Autodesk Inventor part; units mm, degrees
ref_plane "YZ Plane" through (0, 0, 0) normal (1, 0, 0) x (0, 1, 0)
ref_plane "XZ Plane" through (0, 0, 0) normal (0, 1, 0) x (-1, 0, 0)
ref_plane "XY Plane" through (0, 0, 0) normal (0, 0, 1) x (1, 0, 0)
sketch "Sketch1" plane through (0, 0, 0) normal (0, 1, 0) x (-1, 0, 0)
  line L0 (0, 0) -> (0, -650)
  line L1 (0, -650) -> (650, -650)
  line L2 (650, -647) -> (650, -3)
  line L3 (650, 0) -> (0, 0)
  line L4 (0, 0) -> (3, 0)
  line L5 (3, -3) -> (3, -647)
  line L6 (3, -650) -> (0, -650)
  line L7 (0, -650) -> (0, -647)
  line L8 (650, -647) -> (650, -650)
  line L9 (650, -650) -> (647, -650)
  line L10 (647, -647) -> (647, -3)
  line L11 (647, 0) -> (650, 0)
  line L12 (650, 0) -> (650, -3)
  line L13 (0, -3) -> (0, 0)
  line L14 (0, 0) -> (0, -37)
  line L15 (650, -37) -> (650, 0)
  line L16 (650, 0) -> (613, 0)
  line L17 (613, -3) -> (613, -647)
  line L18 (613, -650) -> (650, -650)
  line L19 (650, -650) -> (650, -613)
  line L20 (0, -613) -> (0, -650)
  line L21 (0, -650) -> (37, -650)
  line L22 (37, 0) -> (0, 0)
  line L23 (3, -147.3087) -> (3, -94.9828)
  line L24 (147.3087, -3) -> (94.9828, -3)
  circle A0 centre (16.1109, -108.0348) radius 3
  line L25 (0, -650) -> (3, -650)
  line L26 (0, -647) -> (0, -650)
  line L27 (0, -650) -> (0, -613)
  line L28 (37, -650) -> (0, -650)
  line L29 (3, -502.6913) -> (3, -555.0172)
  line L30 (147.3087, -647) -> (94.9828, -647)
  circle A1 centre (16.1109, -541.9652) radius 3
  line L31 (37, -650) -> (37, -37)
  line L32 (37, -3) -> (37, 0)
  line L33 (650, -3) -> (34.9546, -3)
  line L34 (34.9546, -647) -> (650, -647)
  line L35 (37, -37) -> (0, 0)
  line L36 (37, -613) -> (0, -650)
  line L37 (0, -650) -> (3, -647)
  line L38 (3, -647) -> (3, -3)
  line L39 (3, -3) -> (0, 0)
  line L40 (3, -325) -> (3, -458)
  line L41 (3, -458) -> (20, -458)
  line L42 (3, -325) -> (3, -192)
  line L43 (3, -192) -> (20, -192)
  circle A2 centre (20, -192) radius 3
  circle A3 centre (20, -458) radius 3
  line L44 (647, -3) -> (630, -3)
  line L45 (630, -3) -> (630, -20)
  line L46 (647, -647) -> (630, -647)
  line L47 (630, -647) -> (630, -630)
  circle A4 centre (630, -630) radius 3
  circle A5 centre (630, -20) radius 3
  point P0 (37, -647)
  dimension "d0" = 650
  dimension "d1" = 650
  dimension "d2" = 650
  dimension "d3" = 3
  dimension "d4" = 650
  dimension "d5" = 3
  dimension "d6" = 3
  dimension "d7" = 650
  dimension "d8" = 3
  dimension "d9" = 650
  dimension "d10" = 37
  dimension "d12" = 37
  dimension "d13" = 650
  dimension "d14" = 37
  dimension "d15" = 650
  dimension "d16" = 37
  dimension "d28" = 6
  dimension "d33" = 133
  dimension "d34" = 17
  dimension "d35" = 133
  dimension "d36" = 17
  dimension "d37" = 6
  dimension "d38" = 6
  dimension "d41" = 17
  dimension "d42" = 17
  dimension "d43" = 17
  dimension "d44" = 17
  dimension "d45" = 6
  dimension "d46" = 6
extrude "Extrusion4" add sketch "Sketch1" along normal blind 3 contours L33 L10 L34 L17
extrude "Extrusion5" add sketch "Sketch1" along normal blind 37 contours L2 L34 L10 L33
properties part number "body_inner_center_bar"
Read the model definition and answer for the solid it produces. Units are mm, in the model's axes. A direction names the side the tool comes from. Give positions to 0.01 mm unless a question says otherwise; leave off trailing zeros. Loops run counter-clockwise (first coordinate to the right, second up) from the corner with the lowest first, then second, coordinate; pieces in that order, holes last. Notation, with made-up numbers: M 54.5,44.5 L 89.5,44.5 A21 cw 89.5,70.5 Z; hole C 65,-34.5 d5. An arc over 180 degrees is marked long. Write each question's results on one line, items separated by ' | '.
1. Straight lines are drawn through the part: line 1 (Z direction, x = -630, y = 1); line 2 (X direction, y = 0.8, z = -20); line 3 (X direction, y = 21, z = -111.5). For each, find the intervals that lie inside material, in ascending order. Write a range as [from, to].
Values:
line 1: z = [-647, -633], [-627, -23], [-17, -3] | line 2: x = [-650, -633], [-627, -613] | line 3: x = [-650, -647]
2. Section B-B on y = 29.5 is taken. Give the vertices of the cut face in (x, z), plus the area to 3 significant figures.
Values:
outline: M -650,-647 L -647,-647 L -647,-3 L -650,-3 Z | area: 1,930 mm^2
3. Section A-A on z = -56.5 is taken. Give the vertices of the cut face in (x, y).
Values:
outline: M -650,0 L -613,0 L -613,3 L -647,3 L -647,37 L -650,37 Z
4. A tool of negligible diameter and unlimited length cuts with its end or side. For faces 1 (the face through (-650, 18, -330)), 2 (the face through (-630, 3, -320)), from which of +Z, -Z, +X, -X, +Y, -Y can it reach the whole face along a straight path? Write none if from no direction.
Values:
face 1: +Z, -Z, -X, +Y, -Y | face 2: +Z, -Z, +X, +Y
5. Given pin 1 (1.5 mm diameter, centred on x = -640, z = -497.5, fed in from +Y); pin 2 (5 mm diameter, centred on y = 6.5, z = -190.5, fed in from +X), each flat-ended and moving along its own axis, determine where each tip first touches the part or whether it passes through.
Values:
pin 1: stops at y = 3 | pin 2: stops at x = -647
